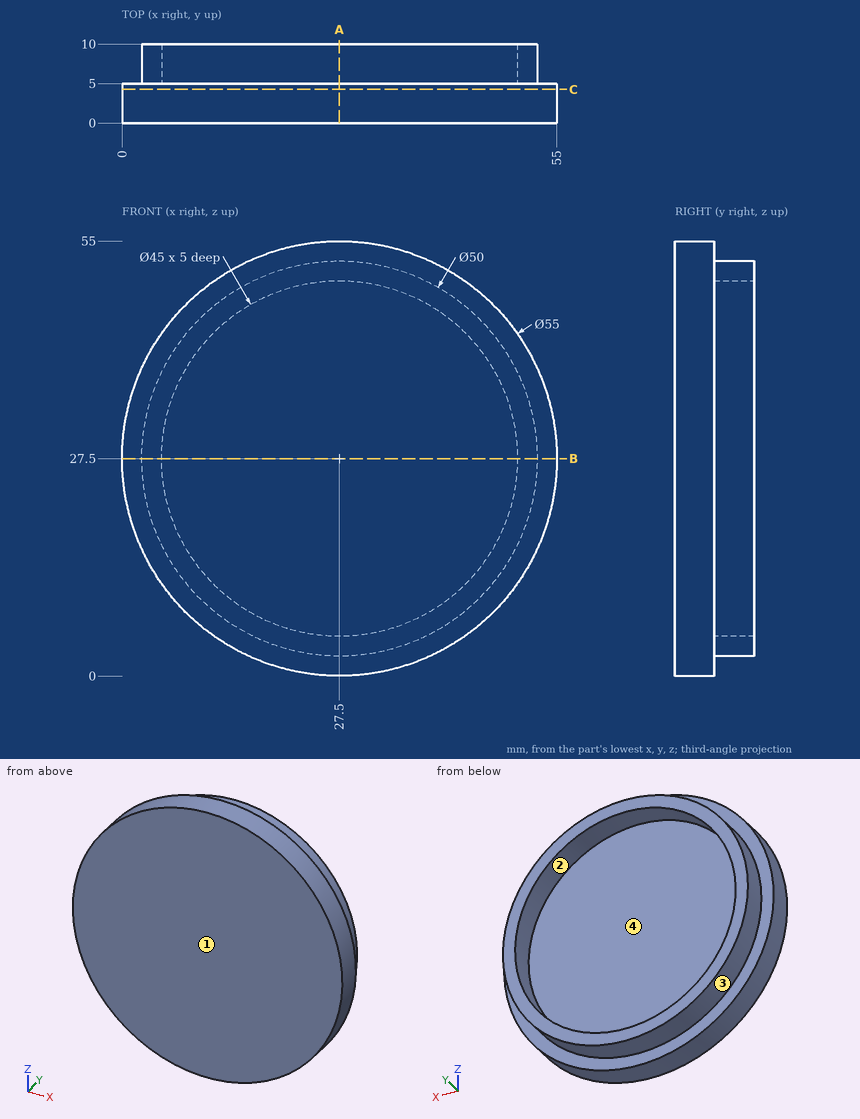
The drawing under review shows one solid part. Ordinate dimensions are in mm from its lowest x, y, z. Coordinates: 2 decimals unless noted, no trailing zeros. Write each loop counter-clockwise with the first axis right and the second up, starting at its lowest first coordinate (ties: lowest second). Pieces come first, ordered by that corner, then holes. Notation, with made-up numbers: (-20, 23.5) - (5, 23.5) arc R30 cw to (5, 59.5) - close; hole circle Ø8 at (58.25, -34.5). An arc over 180 degrees is marked (long way). Put each result on its own line as item: value.
1. Add section A-A, the plane x = 27.5. Give the boundary of the cut face in (y, z).
Values found:
outline: (0, 0) - (5, 0) - (5, 2.5) - (10, 2.5) - (10, 5) - (5, 5) - (5, 50) - (10, 50) - (10, 52.5) - (5, 52.5) - (5, 55) - (0, 55) - close
2. For pin 1 (1 mm diameter, centred on y = 2.5, z = 31.5, fed in from +X); pin 2 (16.5 mm diameter, centred on x = 26, z = 32, fed in from +Y); pin 3 (6 mm diameter, centred on x = 36, y = 7.5, fed in from +Z); pin 4 (3 mm diameter, centred on x = 26, y = 3.5, fed in from -Z), all flat-tipped, find the tip position at first contact; note any pin that passes through.
Values found:
pin 1: x = 54.78
pin 2: y = 5
pin 3: z = 54.14
pin 4: z = 0
3. Add section B-B, the plane z = 27.5. Give the boundary of the cut face in (x, y), then the cut area to 3 significant figures.
Values found:
outline: (0, 0) - (55, 0) - (55, 5) - (52.5, 5) - (52.5, 10) - (50, 10) - (50, 5) - (5, 5) - (5, 10) - (2.5, 10) - (2.5, 5) - (0, 5) - close
area: 300 mm²
4. Mouldability with a two-part tool opening along Z and no side actions: class the marked faces 1, 2, 3 and 4 as released by +Z, released by -Z, zero draft, split by the parting line, or undercut.
Values found:
face 1: zero draft
face 2: undercut
face 3: split by the parting line
face 4: undercut
5. Add section C-C, the plane y = 4.25. Give the boundary of the cut face in (x, z), then the cut area to 3 significant figures.
Values found:
outline: circle Ø55 at (27.5, 27.5)
area: 2,380 mm²
6. Wall thickness on probe 1 along X at (y, z) = (7.8, 27.5); probe 2 along Y at (x, z) = (46, 9); probe 3 along X at (y, z) = (7, 9): over which ranges is each line inside the solid? List them lowest first.
Values found:
probe 1: 2.5 to 5, 50 to 52.5
probe 2: 0 to 5
probe 3: 10.68 to 14.69, 40.31 to 44.32
